```python
from build123d import *

# Parameters (mm, degrees)
BOSS_EXTRUDE1_START  = 65.9
BOSS_EXTRUDE1_DEPTH  = 10.5
BOSS_EXTRUDE2_START  = 65.8
BOSS_EXTRUDE2_DEPTH  = 0.6
CHAMFER1_SIZE        = 3
CHAMFER2_SIZE        = 3
BOSS_EXTRUDE3_START  = 62.7
SKETCH3_W            = 2.3
SKETCH3_H            = 23
BOSS_EXTRUDE3_DEPTH  = 6.6
BOSS_EXTRUDE4_START  = 54.5
SKETCH4_W            = 2.3
SKETCH4_H            = 6.6
BOSS_EXTRUDE4_DEPTH  = 23
BOSS_EXTRUDE5_START  = 65.9
SKETCH5_R            = 4.6
BOSS_EXTRUDE5_DEPTH  = 2.3
BOSS_EXTRUDE6_START  = 75.2
SKETCH6_R            = 6.1
BOSS_EXTRUDE6_DEPTH  = 1.7
BOSS_EXTRUDE7_START  = 68.1
SKETCH7_R            = 3
BOSS_EXTRUDE7_DEPTH  = 7.2
BOSS_EXTRUDE8_START  = 65.1
SKETCH8_W            = 6.1
SKETCH8_H            = 1.1
BOSS_EXTRUDE8_DEPTH  = 1.8
BOSS_EXTRUDE9_START  = 71.5
SKETCH9_W            = 6.1
SKETCH9_H            = 1.8
BOSS_EXTRUDE9_DEPTH  = 1.1
BOSS_EXTRUDE10_START = 65.1
SKETCH10_W           = 6.1
SKETCH10_H           = 1.1
BOSS_EXTRUDE10_DEPTH = 1.8
BOSS_EXTRUDE11_START = 59.4
SKETCH11_W           = 6.1
SKETCH11_H           = 1.8
BOSS_EXTRUDE11_DEPTH = 1.1
BOSS_EXTRUDE12_START = 65.1
SKETCH12_W           = 7.3
SKETCH12_H           = 3.4
BOSS_EXTRUDE12_DEPTH = 1.8
BOSS_EXTRUDE13_START = 72.6
SKETCH13_W           = 7.3
SKETCH13_H           = 1.8
BOSS_EXTRUDE13_DEPTH = 3.4
BOSS_EXTRUDE14_START = 65.1
SKETCH14_W           = 7.3
SKETCH14_H           = 3.4
BOSS_EXTRUDE14_DEPTH = 1.8
BOSS_EXTRUDE15_START = 56
SKETCH15_W           = 7.3
SKETCH15_H           = 1.8
BOSS_EXTRUDE15_DEPTH = 3.4
BOSS_EXTRUDE16_START = 64.4
BOSS_EXTRUDE16_DEPTH = 2.05
BOSS_EXTRUDE17_START = 61.4
SKETCH17_R           = 16.1
SKETCH17_R_2         = 15.2
BOSS_EXTRUDE17_DEPTH = 5.05
BOSS_EXTRUDE18_START = 63
SKETCH18_W           = 3.2
SKETCH18_H           = 4
BOSS_EXTRUDE18_DEPTH = 6
BOSS_EXTRUDE19_START = 26
SKETCH19_W           = 20
SKETCH19_H           = 56
BOSS_EXTRUDE19_DEPTH = 80


with BuildPart() as part:
    # Sketch1 → Boss-Extrude1 (new body)
    with BuildSketch(Plane(origin=(0, 0, 0), x_dir=(0, 0, -1), z_dir=(1, 0, 0)).offset(BOSS_EXTRUDE1_START)):
        with BuildLine():
            Line((-49.657293521, -24.929701405), (-54.04649339, -57.848700423))
            ThreePointArc((-54.04649339, -57.848700423), (-53.234221048, -59.119126346), (-52.95, -60.6))
            Line((-52.95, -60.6), (-52.95, -69.4))
            ThreePointArc((-52.95, -69.4), (-54.121572875, -72.228427125), (-56.95, -73.4))
            Line((-56.95, -73.4), (-85.85, -73.4))
            ThreePointArc((-85.85, -73.4), (-88.678427125, -72.228427125), (-89.85, -69.4))
            Line((-89.85, -69.4), (-89.85, -60.6))
            ThreePointArc((-89.85, -60.6), (-88.678427125, -57.771572875), (-85.85, -56.6))
            Line((-85.85, -56.6), (-78.12, -56.6))
            Line((-78.12, -56.6), (-82.342706479, -24.929701405))
            ThreePointArc((-82.342706479, -24.929701405), (-82.412282932, -24.49821266), (-82.505320186, -24.071167593))
            ThreePointArc((-82.505320186, -24.071167593), (-66, -3), (-49.494679814, -24.071167593))
            ThreePointArc((-49.494679814, -24.071167593), (-49.587717068, -24.49821266), (-49.657293521, -24.929701405))
        make_face()
    extrude(amount=BOSS_EXTRUDE1_DEPTH)


with BuildPart() as body_2:
    # Sketch2 → Boss-Extrude2 (new body)
    with BuildSketch(Plane(origin=(0, 0, 0), x_dir=(0, 0, -1), z_dir=(1, 0, 0)).offset(BOSS_EXTRUDE2_START)):
        with BuildLine():
            Line((-50.450275841, -24.823970429), (-54.893518409, -58.148289686))
            ThreePointArc((-54.893518409, -58.148289686), (-54.049936113, -59.247362039), (-53.75, -60.6))
            Line((-53.75, -60.6), (-53.75, -69.4))
            ThreePointArc((-53.75, -69.4), (-54.6872583, -71.6627417), (-56.95, -72.6))
            Line((-56.95, -72.6), (-85.85, -72.6))
            ThreePointArc((-85.85, -72.6), (-88.1127417, -71.6627417), (-89.05, -69.4))
            Line((-89.05, -69.4), (-89.05, -60.6))
            ThreePointArc((-89.05, -60.6), (-88.1127417, -58.3372583), (-85.85, -57.4))
            Line((-85.85, -57.4), (-77.206253549, -57.4))
            Line((-77.206253549, -57.4), (-81.549724159, -24.823970429))
            ThreePointArc((-81.549724159, -24.823970429), (-81.626258257, -24.34933281), (-81.728599236, -23.879583236))
            ThreePointArc((-81.728599236, -23.879583236), (-66, -3.8), (-50.271400764, -23.879583236))
            ThreePointArc((-50.271400764, -23.879583236), (-50.373741743, -24.34933281), (-50.450275841, -24.823970429))
        make_face()
    extrude(amount=BOSS_EXTRUDE2_DEPTH)


with BuildPart() as part_1:
    add(part.part)

    # Combine1: cut body 2
    add(body_2.part, mode=Mode.SUBTRACT)

    # Chamfer1
    chamfer1_edges = [part_1.edges().sort_by_distance(p)[0] for p in [
        (76.4, -41.389200914, 51.851893455),
        (76.4, -24.49821266, 49.587717068),
        (76.4, -24.49821266, 82.412282932),
        (76.4, -3, 66),
        (76.4, -40.764850703, 80.23135324),
    ]]
    chamfer(chamfer1_edges, length=CHAMFER1_SIZE)

    # Chamfer2
    chamfer2_edges = [part_1.edges().sort_by_distance(p)[0] for p in [
        (76.4, -56.6, 80.471725405),
        (76.4, -57.771572875, 88.678427125),
        (76.4, -57.786965833, 54.106263237),
        (76.4, -65, 89.85),
        (76.4, -65, 52.95),
        (76.4, -72.228427125, 88.678427125),
        (76.4, -72.228427125, 54.121572875),
        (76.4, -73.4, 71.4),
    ]]
    chamfer(chamfer2_edges, length=CHAMFER2_SIZE)


with BuildPart() as body_2_2:
    # Sketch3 → Boss-Extrude3 (new body)
    with BuildSketch(Plane.XY.offset(BOSS_EXTRUDE3_START)):
        with Locations((67.05, -20)):
            Rectangle(SKETCH3_W, SKETCH3_H)
    extrude(amount=BOSS_EXTRUDE3_DEPTH)


with BuildPart() as part_2:
    add(part_1.part)

    # Combine2: cut body 2 2
    add(body_2_2.part, mode=Mode.SUBTRACT)


with BuildPart() as body_2_3:
    # Sketch4 → Boss-Extrude4 (new body)
    with BuildSketch(Plane.XY.offset(BOSS_EXTRUDE4_START)):
        with Locations((67.05, -20)):
            Rectangle(SKETCH4_W, SKETCH4_H)
    extrude(amount=BOSS_EXTRUDE4_DEPTH)


with BuildPart() as part_3:
    add(part_2.part)

    # Combine3: cut body 2 3
    add(body_2_3.part, mode=Mode.SUBTRACT)


with BuildPart() as body_2_4:
    # Sketch5 → Boss-Extrude5 (new body)
    with BuildSketch(Plane(origin=(0, 0, 0), x_dir=(0, 0, -1), z_dir=(1, 0, 0)).offset(BOSS_EXTRUDE5_START)):
        with Locations((-66, -20)):
            Circle(SKETCH5_R)
    extrude(amount=BOSS_EXTRUDE5_DEPTH)


with BuildPart() as part_4:
    add(part_3.part)

    # Combine4: cut body 2 4
    add(body_2_4.part, mode=Mode.SUBTRACT)


with BuildPart() as body_2_5:
    # Sketch6 → Boss-Extrude6 (new body)
    with BuildSketch(Plane(origin=(0, 0, 0), x_dir=(0, 0, -1), z_dir=(1, 0, 0)).offset(BOSS_EXTRUDE6_START)):
        with Locations((-66, -20)):
            Circle(SKETCH6_R)
    extrude(amount=BOSS_EXTRUDE6_DEPTH)


with BuildPart() as part_5:
    add(part_4.part)

    # Combine5: cut body 2 5
    add(body_2_5.part, mode=Mode.SUBTRACT)


with BuildPart() as body_2_6:
    # Sketch7 → Boss-Extrude7 (new body)
    with BuildSketch(Plane(origin=(0, 0, 0), x_dir=(0, 0, -1), z_dir=(1, 0, 0)).offset(BOSS_EXTRUDE7_START)):
        with Locations((-66, -20)):
            Circle(SKETCH7_R)
    extrude(amount=BOSS_EXTRUDE7_DEPTH)


with BuildPart() as part_6:
    add(part_5.part)

    # Combine6: cut body 2 6
    add(body_2_6.part, mode=Mode.SUBTRACT)


with BuildPart() as body_2_7:
    # Sketch8 → Boss-Extrude8 (new body)
    with BuildSketch(Plane.XY.offset(BOSS_EXTRUDE8_START)):
        with Locations((71.15, -13.95)):
            Rectangle(SKETCH8_W, SKETCH8_H)
    extrude(amount=BOSS_EXTRUDE8_DEPTH)


with BuildPart() as part_7:
    add(part_6.part)

    # Combine7: cut body 2 7
    add(body_2_7.part, mode=Mode.SUBTRACT)


with BuildPart() as body_2_8:
    # Sketch9 → Boss-Extrude9 (new body)
    with BuildSketch(Plane.XY.offset(BOSS_EXTRUDE9_START)):
        with Locations((71.15, -20)):
            Rectangle(SKETCH9_W, SKETCH9_H)
    extrude(amount=BOSS_EXTRUDE9_DEPTH)


with BuildPart() as part_8:
    add(part_7.part)

    # Combine8: cut body 2 8
    add(body_2_8.part, mode=Mode.SUBTRACT)


with BuildPart() as body_2_9:
    # Sketch10 → Boss-Extrude10 (new body)
    with BuildSketch(Plane.XY.offset(BOSS_EXTRUDE10_START)):
        with Locations((71.15, -26.05)):
            Rectangle(SKETCH10_W, SKETCH10_H)
    extrude(amount=BOSS_EXTRUDE10_DEPTH)


with BuildPart() as part_9:
    add(part_8.part)

    # Combine9: cut body 2 9
    add(body_2_9.part, mode=Mode.SUBTRACT)


with BuildPart() as body_2_10:
    # Sketch11 → Boss-Extrude11 (new body)
    with BuildSketch(Plane.XY.offset(BOSS_EXTRUDE11_START)):
        with Locations((71.15, -20)):
            Rectangle(SKETCH11_W, SKETCH11_H)
    extrude(amount=BOSS_EXTRUDE11_DEPTH)


with BuildPart() as part_10:
    add(part_9.part)

    # Combine10: cut body 2 10
    add(body_2_10.part, mode=Mode.SUBTRACT)


with BuildPart() as body_2_11:
    # Sketch12 → Boss-Extrude12 (new body)
    with BuildSketch(Plane.XY.offset(BOSS_EXTRUDE12_START)):
        with Locations((71.75, -11.7)):
            Rectangle(SKETCH12_W, SKETCH12_H)
    extrude(amount=BOSS_EXTRUDE12_DEPTH)


with BuildPart() as part_11:
    add(part_10.part)

    # Combine11: cut body 2 11
    add(body_2_11.part, mode=Mode.SUBTRACT)


with BuildPart() as body_2_12:
    # Sketch13 → Boss-Extrude13 (new body)
    with BuildSketch(Plane.XY.offset(BOSS_EXTRUDE13_START)):
        with Locations((71.75, -20)):
            Rectangle(SKETCH13_W, SKETCH13_H)
    extrude(amount=BOSS_EXTRUDE13_DEPTH)


with BuildPart() as part_12:
    add(part_11.part)

    # Combine12: cut body 2 12
    add(body_2_12.part, mode=Mode.SUBTRACT)


with BuildPart() as body_2_13:
    # Sketch14 → Boss-Extrude14 (new body)
    with BuildSketch(Plane.XY.offset(BOSS_EXTRUDE14_START)):
        with Locations((71.75, -28.3)):
            Rectangle(SKETCH14_W, SKETCH14_H)
    extrude(amount=BOSS_EXTRUDE14_DEPTH)


with BuildPart() as part_13:
    add(part_12.part)

    # Combine13: cut body 2 13
    add(body_2_13.part, mode=Mode.SUBTRACT)


with BuildPart() as body_2_14:
    # Sketch15 → Boss-Extrude15 (new body)
    with BuildSketch(Plane.XY.offset(BOSS_EXTRUDE15_START)):
        with Locations((71.75, -20)):
            Rectangle(SKETCH15_W, SKETCH15_H)
    extrude(amount=BOSS_EXTRUDE15_DEPTH)


with BuildPart() as part_14:
    add(part_13.part)

    # Combine14: cut body 2 14
    add(body_2_14.part, mode=Mode.SUBTRACT)

    # Sketch16 → Boss-Extrude16 (add)
    with BuildSketch(Plane(origin=(0, 0, 0), x_dir=(0, 0, -1), z_dir=(1, 0, 0)).offset(BOSS_EXTRUDE16_START)):
        with BuildLine():
            Line((-51.904610688, -14.86969785), (-52.468426261, -15.074909936))
            ThreePointArc((-52.468426261, -15.074909936), (-66, -5.6), (-79.531573739, -15.074909936))
            Line((-79.531573739, -15.074909936), (-80.095389312, -14.86969785))
            ThreePointArc((-80.095389312, -14.86969785), (-66, -5), (-51.904610688, -14.86969785))
        make_face()
    extrude(amount=BOSS_EXTRUDE16_DEPTH)

    # Sketch17 → Boss-Extrude17 (add)
    with BuildSketch(Plane(origin=(0, 0, 0), x_dir=(0, 0, -1), z_dir=(1, 0, 0)).offset(BOSS_EXTRUDE17_START)):
        with Locations((-66, -20)):
            Circle(SKETCH17_R)
        with Locations((-66, -20)):
            Circle(SKETCH17_R_2, mode=Mode.SUBTRACT)
    extrude(amount=BOSS_EXTRUDE17_DEPTH)


with BuildPart() as body_2_15:
    # Sketch18 → Boss-Extrude18 (new body)
    with BuildSketch(Plane.XY.offset(BOSS_EXTRUDE18_START)):
        with Locations((64.8, -36)):
            Rectangle(SKETCH18_W, SKETCH18_H)
    extrude(amount=BOSS_EXTRUDE18_DEPTH)


with BuildPart() as part_15:
    add(part_14.part)

    # Combine15: cut body 2 15
    add(body_2_15.part, mode=Mode.SUBTRACT)


with BuildPart() as body_2_16:
    # Sketch19 → Boss-Extrude19 (new body)
    with BuildSketch(Plane.XY.offset(BOSS_EXTRUDE19_START)):
        with Locations((70, -72)):
            Rectangle(SKETCH19_W, SKETCH19_H)
    extrude(amount=BOSS_EXTRUDE19_DEPTH)


with BuildPart() as part_16:
    add(part_15.part)

    # Combine16: cut body 2 16
    add(body_2_16.part, mode=Mode.SUBTRACT)


solid = part_16.part
```
Design review of the part built by this model. Coordinates are the model's own, in mm. A direction names the side the tool comes from. Give positions to 0.01 mm unless a question says otherwise; leave off trailing zeros. Loops run counter-clockwise (first coordinate to the right, second up) from the corner with the lowest first, then second, coordinate; pieces in that order, holes last. Notation, with made-up numbers: M 19,70.25 L 61,70.25 A17 cw 61,103.25 Z; hole C 63.25,-37 d3. An arc over 180 degrees is marked long. Return JSON: item names as keys, results as strings. Group by question number.
Item 1: We need section C-C (y = -27.5). Give the boundary of the cut face in (x, z), and give its area (3 significant figures).
Item 2: For probe 1 along Z at (x, y) = (71.5, -20); probe 2 along Y at (x, z) = (72.25, 66); probe 3 along Y at (x, z) = (65.3, 66), list the stretches that pass through material, from the lowest coordinate up.
Item 3: Mouldability with a two-part tool opening along Y and no side actions: class faces 1 (the flat face through (69.6, -34.33, 50.91)), 2 (the flat face through (75, -20, 72.6)), 3 (the flat face through (63.2, -35.5, 66)), 4 (the flat face through (67, -23.3, 73)) as released by +Y, released by -Y, zero draft, split by the parting line, or undercut.
Item 4: We need section B-B (z = 66). Give the number of separate pieces and of enclosed holes in the cut face, and give its area (3 significant figures).
Item 5: Insertion check: pin 1 Ø2 at (x, y) = (67.5, -13.5) entering from -Z; pin 2 Ø6 at (x, y) = (66, -34.5) entering from +Z; pin 3 Ø0.5 at (y, z) = (-28.5, 65.5) entering from -X. Each pin has a flat end and moves straight along its axis. Give the tip position at first contact, or say it passes through.
Item 6: Tool access review of faces 5 (the flat face through (64.8, -35.4, 69)), 6 (the cylindrical face through (63.865, -9.727, 77.203)), 7 (the cylindrical face through (69.598, -24.492, 49.587)): name each direction out of +Z, -Z, +X, -X, +Y, -Y from which nothing blocks a thin tool from reaching the whole face with its end or side.
Item 7: We need section D-D (x = 74.75). Give the boundary of the cut face in (y, z).
Item 8: We need section A-A (x = 67). Give the boundary of the cut face in (y, z), and give its area (3 significant figures).
Output:
{
 "1": {"outline": "M 61.4,51.75 L 66.4,51.75 L 66.4,50.81 L 65.9,50.81 L 65.9,50 L 73.4,50 L 76.4,53.03 L 76.4,78.97 L 73.4,82 L 65.9,82 L 65.9,81.19 L 66.4,81.19 L 66.4,80.25 L 61.4,80.25 L 61.4,79.22 L 66.4,79.22 L 66.4,69.3 L 68.2,69.3 L 68.2,66.9 L 75.4,66.9 L 75.4,65.1 L 68.2,65.1 L 68.2,62.7 L 66.4,62.7 L 66.4,52.78 L 61.4,52.78 Z", "area": "297 mm^2"},
 "2": {"probe 1": "z = 49 to 56, 60.5 to 63, 69 to 71.5, 76 to 83", "probe 2": "y = -44 to -30, -25.5 to -23, -17 to -14.5, -10 to -3", "probe 3": "y = -5.6 to -5, -4.8 to -3.9"},
 "3": {"face 1": "released by -Y", "face 2": "undercut", "face 3": "zero draft", "face 4": "undercut"},
 "4": {"separate pieces": "3", "enclosed holes": "0", "area": "253 mm^2"},
 "5": {"pin 1": "stops at z = 49.91", "pin 2": "stops at z = 81.47", "pin 3": "stops at x = 75.4"},
 "6": {"face 5": "-Y", "face 6": "-X", "face 7": "-Z, +X, -X, -Y"},
 "7": {"outline": "M -44,53.56 L -24.75,51 A9.35 cw -23.75,50.81 A15.65 ccw long -23.75,81.19 A9.35 cw -24.75,81 L -44,78.44 Z; hole M -30,65.1 L -26.6,65.1 L -26.6,66.9 L -30,66.9 Z; hole C -20,66 d6; hole M -20.9,56 L -19.1,56 L -19.1,59.4 L -20.9,59.4 Z; hole M -20.9,72.6 L -19.1,72.6 L -19.1,76 L -20.9,76 Z; hole M -13.4,65.1 L -10,65.1 L -10,66.9 L -13.4,66.9 Z"},
 "8": {"outline": "M -44,52.2 L -24.93,49.66 A8 cw -24.07,49.49 A17 ccw long -24.07,82.51 A8 cw -24.93,82.34 L -44,79.8 Z; hole M -31.5,62.7 L -23.3,62.7 L -23.3,54.5 L -16.7,54.5 L -16.7,62.7 L -8.5,62.7 L -8.5,69.3 L -16.7,69.3 L -16.7,77.5 L -23.3,77.5 L -23.3,69.3 L -31.5,69.3 Z", "area": "934 mm^2"}
}
